Autodesk Fusion 360 part; units mm, degrees
sketch "Sketch1" plane through (0, 0, 0) normal (0, 1, 0) x (1, 0, 0)
  line L0 (-30, -70) -> (50, -70)
  line L1 (70, -50) -> (70, -20)
  line L2 (70, -20) -> (-50, -20)
  line L3 (-50, -20) -> (-50, -50)
  arc A0 (50, -70) -> (70, -50) centre (50, -50) ccw
  arc A1 (-50, -50) -> (-30, -70) centre (-30, -50) ccw
  point P0 (-50, -70)
  point P1 (70, -70)
  dimension "d1" = 120
  dimension "d2" = 50
  dimension "d3" = 20
  dimension "d4" = 20
extrude "Extrude1" add sketch "Sketch1" along normal blind 20
sketch "Sketch2" plane through (0, 0, 0) normal (0, -1, 0) x (1, 0, 0)
  arc A0 (-30, 70) -> (-50, 50) centre (-30, 50) ccw
  line L0 (-50, 50) -> (-50, 20)
  line L1 (-50, 20) -> (70, 20)
  line L2 (70, 20) -> (70, 50)
  arc A1 (70, 50) -> (50, 70) centre (50, 50) ccw
  line L3 (50, 70) -> (-30, 70)
  line L4 (-30, 44) -> (50, 44)
  arc A2 (50, 44) -> (50, 56) centre (50, 50) ccw
  line L5 (50, 56) -> (-30, 56)
  arc A3 (-30, 56) -> (-30, 44) centre (-30, 50) ccw
  line L6 (-30, 50) -> (50, 50) construction
  dimension "d7" = 12
extrude "Extrude2" cut sketch "Sketch2" against normal blind 120 contours L4 A2 L5 A3
sketch "Sketch3" plane through (-50, 0, 0) normal (-1, 0, 0) x (0, -1, 0)
  line L0 (0, 20) -> (0, 50)
  line L1 (0, 50) -> (-20, 50)
  line L2 (-20, 50) -> (-20, 20)
  line L3 (-20, 20) -> (0, 20)
  line L4 (-20, 20) -> (80, 20)
  line L5 (80, 20) -> (80, 40)
  line L6 (80, 40) -> (-20, 40)
  line L7 (-20, 40) -> (-20, 20)
  dimension "d13" = 100
  dimension "d14" = 20
extrude "Extrude3" add sketch "Sketch3" against normal blind 120 contours L0 L4 L5 L6
fillet "Fillet1" radius 30 1 edges at (-50, -80, 30)
fillet "Fillet2" radius 30 1 edges at (70, -80, 30)
sketch "Sketch4" plane through (0, 0, 40) normal (0, 0, 1) x (-1, 0, 0)
  arc A0 (-40, 80) -> (-70, 50) centre (-40, 50) ccw
  line L0 (-70, 50) -> (-70, 0)
  line L1 (-70, 0) -> (50, 0)
  line L2 (50, 0) -> (50, 50)
  arc A1 (50, 50) -> (20, 80) centre (20, 50) ccw
  line L3 (20, 80) -> (-40, 80)
  line L4 (20, 52.1541) -> (-40, 52.1541)
  arc A2 (-40, 52.1541) -> (-40, 22.1541) centre (-40, 37.1541) ccw
  line L5 (-40, 22.1541) -> (20, 22.1541)
  arc A3 (20, 22.1541) -> (20, 52.1541) centre (20, 37.1541) ccw
  line L6 (20, 37.1541) -> (-40, 37.1541) construction
  dimension "d21" = 30
  dimension "d24" = 30
extrude "Extrude4" cut sketch "Sketch4" against normal blind 80 contours L4 A2 L5 A3
CAD build for the part. Positions are in the model's coordinates, mm. A direction names the side the tool comes from. Give positions to 0.01 mm unless a question says otherwise; leave off trailing zeros. Order: outer loops, then holes, each group sorted by start corner. A loop starts at its lowest first (then second) coordinate and runs counter-clockwise, first axis right, second up. Notation, with made-up numbers: (47, 47.25) - (55, 47.25) arc R21 cw to (55, 76.25) - close; hole circle Ø9 at (7, 87). An arc over 180 degrees is marked (long way). Answer in a Markdown table with one row per item.
1. Saw through at A-A, the plane x = 17. Give the cut face in (y, z), plus the area to 3 significant figures.
Data:
| item | result |
|---|---|
| outline | (-80, 20) - (-52.15, 20) - (-52.15, 40) - (-80, 40) - close; (-22.15, 20) - (20, 20) - (20, 44) - (0, 44) - (0, 40) - (-22.15, 40) - close; (0, 56) - (20, 56) - (20, 70) - (0, 70) - close |
| area | 1,760 mm² |
2. Flat gauge pins, fed straight in: pin 1 (15 mm diameter, centred on x = 26.5, z = 61, fed in from -Y); pin 2 (10 mm diameter, centred on y = -66, z = 41, fed in from -X); pin 3 (12 mm diameter, centred on y = -60.5, z = 50.5, fed in from -X); pin 4 (3 mm diameter, centred on x = -13, y = -10.5, fed in from +Z). Where does each tip first touch, or does it go through?
Data:
| item | result |
|---|---|
| pin 1 | stops at y = 0 |
| pin 2 | stops at x = -47.87 |
| pin 3 | passes through |
| pin 4 | stops at z = 40 |
3. Saw through at B-B, the plane z = 24.5. Give the cut face in (x, y).
Data:
| item | result |
|---|---|
| outline | (-50, -50) arc R30 ccw to (-20, -80) - (40, -80) arc R30 ccw to (70, -50) - (70, 20) - (-50, 20) - close; hole (-20, -52.15) - (40, -52.15) arc R15 ccw to (40, -22.15) - (-20, -22.15) arc R15 ccw to start |
4. Probe probe 1 along Z at (x, y) = (15.5, 14); probe 2 along Y at (x, z) = (29, 35.5); probe 3 along Z at (x, y) = (-7, -22). List the from-to ranges inside material, lowest first. Write a range as [from, to].
Data:
| item | result |
|---|---|
| probe 1 | z = [20, 44], [56, 70] |
| probe 2 | y = [-80, -52.15], [-22.15, 20] |
| probe 3 | z = [20, 40] |
5. Saw through at C-C, the plane x = 59.5. Give the cut face in (y, z), plus the area to 3 significant figures.
Data:
| item | result |
|---|---|
| outline | (-72.8, 20) - (20, 20) - (20, 67.6) - (0, 67.6) - (0, 40) - (-72.8, 40) - close |
| area | 2,410 mm² |
6. Tool access for faces 1 (the cylindrical face through (60.979, -71.445, 30.14)), 2 (the flat face through (10, -52.154, 30)), 3 (the cylindrical face through (56, 10, 50)), 4 (the flat face through (9, -58, 40)): list every direction of +Z, -Z, +X, -X, +Y, -Y with a clear straight run to the whole face (end or side of a thin tool).
Data:
| item | result |
|---|---|
| face 1 | +Z, -Z, +X, -Y |
| face 2 | +Z, -Z |
| face 3 | +Y, -Y |
| face 4 | +Z, +X, -X, -Y |
7. Pull direction Y, two halves, no side cores. Call faces 5 (the flat face through (9, 20, 39)), 6 (the cylindrical face through (55, -37, 30)), 7 (the cylindrical face through (64.297, 9.86, 63.986)), 8 (the flat face through (10, -22.154, 30)): pulls with the +Y half, pulls with the -Y half, needs draft (parallel to the pull), parting line crosses it, or undercut.
Data:
| item | result |
|---|---|
| face 5 | pulls with the +Y half |
| face 6 | undercut |
| face 7 | needs draft |
| face 8 | undercut |
